Build history of the part. All positions in model axes, mm. Face numbers are marked on the shaded views. A direction names the side the tool comes from. Give positions to 0.01 mm unless a question says otherwise; leave off trailing zeros. Order: outer loops, then holes, each group sorted by start corner. A loop starts at its lowest first (then second) coordinate and runs counter-clockwise, first axis right, second up. Notation, with made-up numbers: M 68,19.5 L 82,19.5 A25 cw 82,36.5 Z; hole C 89,-30 d4. An arc over 180 degrees is marked long. One line per item, written item: value.
from build123d import *

# Parameters (mm, degrees)
ESBO_O1_W                = 26
ESBO_O1_H                = 20
RESSALTO_EXTRUS_O1_DEPTH = 6
ESBO_O2_W                = 2
ESBO_O2_H                = 20
RESSALTO_EXTRUS_O2_DEPTH = 4
CORTE_EXTRUS_O1_DEPTH    = 2


with BuildPart() as part:
    # Esboço1 → Ressalto-extrusão1 (new body)
    with BuildSketch(Plane.XY):
        with Locations((-13, 10)):
            Rectangle(ESBO_O1_W, ESBO_O1_H)
    extrude(amount=RESSALTO_EXTRUS_O1_DEPTH)

    # Esboço2 → Ressalto-extrusão2 (add)
    with BuildSketch(Plane(origin=(0, 0, 0), x_dir=(-1, 0, 0), z_dir=(0, 0, -1))):
        with Locations((1, 10)):
            Rectangle(ESBO_O2_W, ESBO_O2_H)
    extrude(amount=RESSALTO_EXTRUS_O2_DEPTH)

    # Esboço3 → Corte-extrusão1 (cut)
    with BuildSketch(Plane(origin=(0, 0, 0), x_dir=(-1, 0, 0), z_dir=(0, 0, -1))):
        with BuildLine():
            Line((5, 10), (26, 10))
            Line((26, 10), (26, 14))
            Line((26, 14), (5, 14))
            ThreePointArc((5, 14), (3, 12), (5, 10))
        make_face()
    extrude(amount=-CORTE_EXTRUS_O1_DEPTH, mode=Mode.SUBTRACT)


solid = part.part
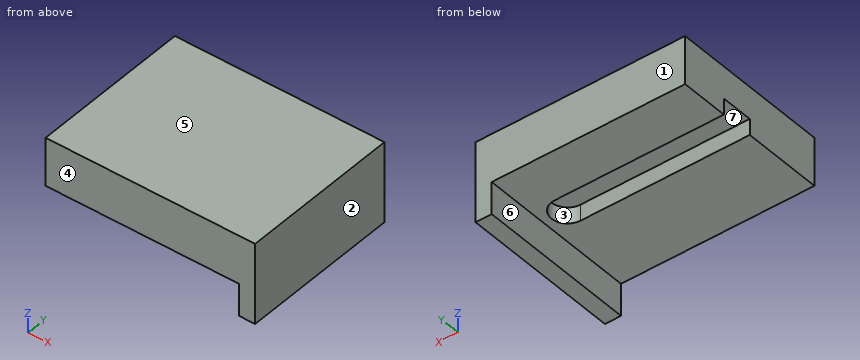
1) Pin check, flat tips, straight feed: pin 1 (8 mm diameter, centred on x = -21.5, y = 17, fed in from -Z); pin 2 (2 mm diameter, centred on y = 9, z = -1.5, fed in from -X). Stop position of each tip, or through.
Check values:
pin 1: z = 0
pin 2: x = -2
2) Tool access for the marked faces 5, 6 and 7: list every direction of +Z, -Z, +X, -X, +Y, -Y with a clear straight run to the whole face (end or side of a thin tool).
Check values:
face 5: +Z, +X, -X, +Y, -Y
face 6: -Z, -X, +Y, -Y
face 7: -Z, -X
3) Saw through at A-A, the plane y = 3.75. Write the cut outline in (x, z).
Check values:
outline: M -26,0 L -2,0 L -2,-4 L 0,-4 L 0,6 L -26,6 Z
4) Saw through at B-B, the plane x = -19.5. Write the cut outline in (y, z), then the cut area to 3 significant figures.
Check values:
outline: M 0,0 L 10,0 L 10,2 L 14,2 L 14,0 L 20,0 L 20,6 L 0,6 Z
area: 112 mm^2
5) Mould opens along Y. For the marked faces 1, 2, 3 and 4 say: released by +Y, released by -Y, zero draft, split by the parting line, or undercut.
Check values:
face 1: released by +Y
face 2: zero draft
face 3: undercut
face 4: released by -Y
6) Saw through at D-D, the plane z = -0.75. Write the cut outline in (x, y).
Check values:
outline: M -2,0 L 0,0 L 0,20 L -2,20 Z
7) Saw through at C-C, the plane z = 1.25. Write the cut outline in (x, y).
Check values:
outline: M -26,0 L 0,0 L 0,20 L -26,20 L -26,14 L -5,14 A2 cw -5,10 L -26,10 Z
8) Drill centre lines: probe 1 along Y at (x, z) = (-20.5, 1.25); probe 2 along X at (y, z) = (16.25, -0.75); probe 3 along Z at (x, y) = (-22, 10.75). Where is each one in solid material? Low to high. Write a range as from..to.
Check values:
probe 1: 0..10, 14..20
probe 2: -2..0
probe 3: 2..6
